Can you work these out from the model? Positions are in its coordinate system, mm. A direction names the side the tool comes from. Round coordinates to 2 decimals unless told otherwise and drop trailing zeros. Loops run counter-clockwise (first coordinate to the right, second up) from the corner with the lowest first, then second, coordinate; pieces in that order, holes last. Notation, with made-up numbers: (73, 83.5) - (130, 83.5) arc R3 ccw to (130, 88.5) - close; hole circle Ø11 at (-14, 70.25). An arc over 180 degrees is marked (long way). Answer as CSV lines item,"result".
Autodesk Fusion 360 part; units mm, degrees
sketch "Sketch1" plane through (0, 0, 0) normal (0, 0, 1) x (1, 0, 0)
  line L0 (-25.4, 25.4) -> (25.4, 25.4)
  line L1 (25.4, 25.4) -> (25.4, -25.4)
  line L2 (25.4, -25.4) -> (-25.4, -25.4)
  line L3 (-25.4, -25.4) -> (-25.4, 25.4)
  line L4 (-25.4, 25.4) -> (25.4, -25.4) construction
  line L5 (25.4, 25.4) -> (-25.4, -25.4) construction
  dimension "d1" = 50.8
  dimension "d2" = 50.8
extrude "Extrude1" add sketch "Sketch1" along normal blind 38.1
sketch "Sketch2" plane through (0, 0, 38.1) normal (0, 0, 1) x (-1, 0, 0)
  line L0 (25.4, 25.4) -> (-25.4, 25.4)
  line L1 (-25.4, 25.4) -> (-25.4, -25.4)
  line L2 (-25.4, -25.4) -> (25.4, -25.4)
  line L3 (25.4, -25.4) -> (25.4, 25.4)
  line L4 (5.08, -5.08) -> (-5.08, -5.08)
  line L5 (-5.08, -5.08) -> (-5.08, 5.08)
  line L6 (-5.08, 5.08) -> (5.08, 5.08)
  line L7 (5.08, 5.08) -> (5.08, -5.08)
  line L8 (5.08, -5.08) -> (-5.08, 5.08) construction
  line L9 (-5.08, -5.08) -> (5.08, 5.08) construction
  line L10 (-25.4, -25.4) -> (25.4, -25.4)
  line L11 (25.4, 25.4) -> (25.4, -25.4)
  line L12 (25.4, 25.4) -> (-25.4, 25.4)
  line L13 (-25.4, -25.4) -> (-25.4, 25.4)
  dimension "d5" = 10.16
  dimension "d6" = 10.16
extrude "Extrude2" cut sketch "Sketch2" against normal blind 7.62
sketch "Sketch3" plane through (0, 0, 30.48) normal (0, 0, 1) x (-1, 0, 0)
  line L0 (-5.08, 5.08) -> (5.08, 5.08)
  line L1 (5.08, 5.08) -> (5.08, -5.08)
  line L2 (5.08, -5.08) -> (-5.08, -5.08)
  line L3 (-5.08, -5.08) -> (-5.08, 5.08)
  line L4 (25.4, 25.4) -> (-25.4, 25.4)
  line L5 (-25.4, 25.4) -> (-25.4, -25.4)
  line L6 (-25.4, -25.4) -> (25.4, -25.4)
  line L7 (25.4, -25.4) -> (25.4, 25.4)
  circle A0 centre (20.32, 20.32) radius 2.032
  circle A1 centre (-20.32, 20.32) radius 2.032
  circle A2 centre (-20.32, -20.32) radius 2.032
  circle A3 centre (20.32, -20.32) radius 2.032
  dimension "d11" = 4.064
  dimension "d13" = 360
  dimension "d14" = 5.08
  dimension "d15" = 5.08
  dimension "d17" = 5.08
  dimension "d18" = 5.08
  dimension "d19" = 5.08
extrude "Extrude3" cut sketch "Sketch3" against normal blind 2.54 contours A0 | A1 | A2 | A3
sketch "Sketch4" plane through (0, 0, 30.48) normal (0, 0, 1) x (-1, 0, 0)
  circle A0 centre (-20.32, 20.32) radius 2.032
  circle A1 centre (20.32, 20.32) radius 2.032
  circle A2 centre (-20.32, -20.32) radius 2.032
  circle A3 centre (20.32, -20.32) radius 2.032
  line L0 (-5.08, 5.08) -> (5.08, 5.08)
  line L1 (5.08, 5.08) -> (5.08, -5.08)
  line L2 (5.08, -5.08) -> (-5.08, -5.08)
  line L3 (-5.08, -5.08) -> (-5.08, 5.08)
  line L4 (25.4, 25.4) -> (-25.4, 25.4)
  line L5 (-25.4, 25.4) -> (-25.4, -25.4)
  line L6 (-25.4, -25.4) -> (25.4, -25.4)
  line L7 (25.4, -25.4) -> (25.4, 25.4)
  circle A4 centre (20.32, -20.32) radius 1.524
  circle A5 centre (20.32, 20.32) radius 1.524
  circle A6 centre (-20.32, 20.32) radius 1.524
  circle A7 centre (-20.32, -20.32) radius 1.524
  dimension "d22" = 3.048
  dimension "d24" = 360
extrude "Extrude4" cut sketch "Sketch4" against normal blind 20.32 contours A4 | A5 | A6 | A7
chamfer "Chamfer1" distance 1.27 angle 45 4 edges at (0, -25.4, 30.48) (25.4, 0, 30.48) (0, 25.4, 30.48) (-25.4, 0, 30.48)
Q1. I'm going to push flat-ended pins straight in: pin 1 Ø1.2 at (x, y) = (21, 20) entering from +Z; pin 2 Ø12 at (x, y) = (-1, 7) entering from +Z; pin 3 Ø3.5 at (x, y) = (21, 20.5) entering from +Z; pin 4 Ø3.5 at (x, y) = (-20.32, 20.32) entering from +Z. Where does each tip first touch, or does it pass through?
Checks:
pin 1,"z = 10.16"
pin 2,"z = 38.1"
pin 3,"z = 30.48"
pin 4,"z = 27.94"
Q2. Imagine slicing it at A-A (x = -0.5). Write out the boundary of the cut face in (y, z).
Checks:
outline,"(-25.4, 0) - (25.4, 0) - (25.4, 29.21) - (24.13, 30.48) - (5.08, 30.48) - (5.08, 38.1) - (-5.08, 38.1) - (-5.08, 30.48) - (-24.13, 30.48) - (-25.4, 29.21) - close"
Q3. We'd pull the mould along Y, two halves only. Please class faces 1 (the flat face through (0, -5.08, 34)), 2 (the flat face through (22, 20, 27.94)), 3 (the flat face through (0, 0, 38.1)): pulls with the +Y half, pulls with the -Y half, needs draft (parallel to the pull), parting line crosses it, or undercut.
Checks:
face 1,"pulls with the -Y half"
face 2,"undercut"
face 3,"needs draft"
Q4. On a 3-axis mill with a long thin cutter (end or side, diameter ignored), from which of +Z, -Z, +X, -X, +Y, -Y can I reach the whole of each face in a straight line? I mean faces 4 (the flat face through (0, 5.08, 34)), 5 (the flat face through (20, -22, 27.94)), 6 (the flat face through (-5.08, 0, 34)), 7 (the flat face through (25.4, 0, 14)). Say none if no direction works.
Checks:
face 4,"+Z, +X, -X, +Y"
face 5,"+Z"
face 6,"+Z, -X, +Y, -Y"
face 7,"+Z, -Z, +X, +Y, -Y"
Q5. Imagine slicing it at C-C (x = -20.32). Write out the boundary of the cut face in (y, z), then the cut area to 3 significant figures.
Checks:
outline,"(-25.4, 0) - (25.4, 0) - (25.4, 29.21) - (24.13, 30.48) - (22.35, 30.48) - (22.35, 27.94) - (21.84, 27.94) - (21.84, 10.16) - (18.8, 10.16) - (18.8, 27.94) - (18.29, 27.94) - (18.29, 30.48) - (-18.29, 30.48) - (-18.29, 27.94) - (-18.8, 27.94) - (-18.8, 10.16) - (-21.84, 10.16) - (-21.84, 27.94) - (-22.35, 27.94) - (-22.35, 30.48) - (-24.13, 30.48) - (-25.4, 29.21) - close"
area,"1,420 mm²"
Q6. If I drill on line 1 along Y through (x, z) = (20.32, 29); line 2 along X through (y, z) = (-20.32, 18.75), over which ranges is the centre line in solid material (lowest first)? Write a range as [from, to].
Checks:
line 1,"[-25.4, -22.35], [-18.29, 18.29], [22.35, 25.4]"
line 2,"[-25.4, -21.84], [-18.8, 18.8], [21.84, 25.4]"
Q7. Imagine slicing it at D-D (z = 33.5). Write out the boundary of the cut face in (x, y), then the cut area to 3 significant figures.
Checks:
outline,"(-5.08, -5.08) - (5.08, -5.08) - (5.08, 5.08) - (-5.08, 5.08) - close"
area,"103 mm²"
